Here's how the part is built. I have some questions about the finished solid (model axes, mm). A direction names the side the tool comes from. Give positions to 0.01 mm unless a question says otherwise; leave off trailing zeros. Write each loop counter-clockwise with the first axis right and the second up, starting at its lowest first coordinate (ties: lowest second). Pieces come first, ordered by that corner, then holes. Notation, with made-up numbers: (42.25, -34) - (57.25, -34) arc R28 ccw to (57.25, -11) - close; hole circle Ø11 at (-37.75, 27.25). An arc over 180 degrees is marked (long way). Use a Markdown table: item, result.
```python
from build123d import *

# Parameters (mm, degrees)
F1_DEPTH = 1520
F2_R     = 9
F2_R_2   = 12
F3_DEPTH = 180


with BuildPart() as f1:
    # F0 (on Front) → F1 (new body)
    with BuildSketch(Plane.XZ):
        with BuildLine():
            Line((-180, 0), (0, 0))
            Line((0, 0), (0, 75))
            Line((0, 75), (-11, 75))
            Line((-11, 75), (-11, 18))
            ThreePointArc((-11, 18), (-14.514719, 9.514719), (-23, 6))
            Line((-23, 6), (-157, 6))
            ThreePointArc((-157, 6), (-165.485281, 9.514719), (-169, 18))
            Line((-169, 18), (-169, 75))
            Line((-169, 75), (-180, 75))
            Line((-180, 75), (-180, 0))
        make_face()
    extrude(amount=-F1_DEPTH)

    # F2 (on face) → F3 (cut)
    with BuildSketch(Plane.YZ):
        with Locations((910, 37.5)):
            Circle(F2_R)
        with Locations((610, 37.5)):
            Circle(F2_R_2)
    extrude(amount=-F3_DEPTH, mode=Mode.SUBTRACT)


solid = f1.part
```
Item 1: If we section it at A-A, the plane z = 62.5: Write out the boundary of the cut face in (x, y).
Values:
| item | result |
|---|---|
| outline | (-180, 0) - (-169, 0) - (-169, 1520) - (-180, 1520) - close; (-11, 0) - (0, 0) - (0, 1520) - (-11, 1520) - close |
Item 2: I need wall thicknesses on line 1 along Y through (x, z) = (-3, 37); line 2 along X through (y, z) = (964.5, 71.5); line 3 along Z through (x, y) = (-174, 610). Which ranges of each line are inside material? Lowest first, please. Write a range as [from, to].
Values:
| item | result |
|---|---|
| line 1 | y = [0, 598.01], [621.99, 901.01], [918.99, 1520] |
| line 2 | x = [-180, -169], [-11, 0] |
| line 3 | z = [0, 25.5], [49.5, 75] |
Item 3: For faces 4 (the flat face through (-11, 749, 47)), 5 (the flat face through (-91, 749, 0)), which set-ups out of +Z, -Z, +X, -X, +Y, -Y let a thin tool reach every point of the face, with its end or its side?
Values:
| item | result |
|---|---|
| face 4 | +Z, +Y, -Y |
| face 5 | -Z, +X, -X, +Y, -Y |
Item 4: If we section it at B-B, the plane y = 1201.5: Write out the boundary of the cut face in (x, z).
Values:
| item | result |
|---|---|
| outline | (-180, 0) - (0, 0) - (0, 75) - (-11, 75) - (-11, 18) arc R12 cw to (-23, 6) - (-157, 6) arc R12 cw to (-169, 18) - (-169, 75) - (-180, 75) - close |
Item 5: If we section it at C-C, the plane x = -76.5: Write out the boundary of the cut face in (y, z).
Values:
| item | result |
|---|---|
| outline | (0, 0) - (1520, 0) - (1520, 6) - (0, 6) - close |
Item 6: Will these pins go through, and if not, where does the flat tip stop? pin 1 Ø23.5 at (y, z) = (910, 37.5) entering from +X; pin 2 Ø12 at (x, y) = (-134, 1029.5) entering from +Z.
Values:
| item | result |
|---|---|
| pin 1 | stops at x = 0 |
| pin 2 | stops at z = 6 |
Item 7: Thinking about a two-plate mould opening in Z: for faces 1 (the cylindrical face through (-174.423, 621.446, 41.104)), 2 (the flat face through (-89, 749, 6)), 3 (the flat face through (-169, 749, 46)), which applies, +Z half, -Z half, draft (parallel to the pull), parting line (faces both ways), or undercut?
Values:
| item | result |
|---|---|
| face 1 | undercut |
| face 2 | +Z half |
| face 3 | draft |
